The listing builds one solid part. Answer for the finished solid, in the listing's coordinates (mm). A direction names the side the tool comes from. Coordinates: 2 decimals unless noted, no trailing zeros. Order: outer loops, then holes, each group sorted by start corner. A loop starts at its lowest first (then second) coordinate and runs counter-clockwise, first axis right, second up. Notation, with made-up numbers: (68.5, -1) -> (119.5, -1) arc R5 cw to (119.5, 4) -> close; hole circle Ø8 at (70.5, 42.25). An arc over 180 degrees is marked (long way). Answer in a Markdown table with one row per item.
```python
from build123d import *

# Parameters (mm, degrees)
BOSS_EXTRUDE1_DEPTH = 11
CHAMFER1_SIZE       = 0.325


with BuildPart() as part:
    # Sketch1 → Boss-Extrude1 (new body)
    with BuildSketch(Plane(origin=(0, 0, 0), x_dir=(0, -1, 0), z_dir=(-1, 0, 0))):
        Polygon((2.886751346, 0), (1.443375673, 2.5), (-1.443375673, 2.5), (-2.886751346, 0), (-1.443375673, -2.5), (1.443375673, -2.5), align=None)
    extrude(amount=-BOSS_EXTRUDE1_DEPTH)

    # Sketch2 → Cut-Revolve1 (revolve, cut)
    with BuildSketch(Plane.XY, mode=Mode.PRIVATE) as cut_revolve1_sk:
        Polygon((0, 1.229375), (0, 0), (9.999979987, 0), (9.2902, 1.229375), (8.270625, 1.229375), (8, 1.5), (8, 1.229375), align=None)
    revolve(cut_revolve1_sk.sketch.rotate(Axis((0, 0, 0), (1, 0, 0)), 270), axis=Axis((0, 0, 0), (1, 0, 0)), mode=Mode.SUBTRACT)

    # Sketch3 → Revolve1 (revolve)
    with BuildSketch(Plane(origin=(0, 0, 0), x_dir=(-1, 0, 0), z_dir=(0, 0, -1)), mode=Mode.PRIVATE) as revolve1_sk:
        Polygon((-17, 1.5), (-17, 0), (-11, 0), (-11, 1.175), (-12.2, 1.175), (-12.2, 1.5), align=None)
    revolve(revolve1_sk.sketch.rotate(Axis((17, 0, 0), (-1, 0, 0)), 270), axis=Axis((17, 0, 0), (-1, 0, 0)))

    # Chamfer1
    chamfer1_edges = [part.edges().sort_by_distance(p)[0] for p in [
        (0, 0, 1.229375),
        (17, 0, -1.5),
    ]]
    chamfer(chamfer1_edges, length=CHAMFER1_SIZE)


solid = part.part
```
(1) Which of the six approach directions +Z, -Z, +X, -X, +Y, -Y give full straight-line access (tool end or side, diameter ignored) to faces 1 (the cylindrical face through (4.11, 1.22, 0.16)), 2 (the flat face through (11, -1, 1)), 3 (the flat face through (17, 0, 0)), 4 (the cylindrical face through (14.47, 0.45, 1.43))?
Check values:
| item | result |
|---|---|
| face 1 | -X |
| face 2 | none |
| face 3 | +Z, -Z, +X, +Y, -Y |
| face 4 | +X |
(2) A cutting plane is placed at A-A, the plane x = 3.5. Determine the outline of the cut face in (y, z), then the cut area to 3 significant figures.
Check values:
| item | result |
|---|---|
| outline | (-2.89, 0) -> (-1.44, -2.5) -> (1.44, -2.5) -> (2.89, 0) -> (1.44, 2.5) -> (-1.44, 2.5) -> close; hole circle Ø2.46 at (0, 0) |
| area | 16.9 mm² |
(3) A cutting plane is placed at B-B, the plane x = 10.25. Determine the outline of the cut face in (y, z), then the cut area to 3 significant figures.
Check values:
| item | result |
|---|---|
| outline | (-2.89, 0) -> (-1.44, -2.5) -> (1.44, -2.5) -> (2.89, 0) -> (1.44, 2.5) -> (-1.44, 2.5) -> close |
| area | 21.7 mm² |
(4) Find the intervals of material crossed by line 1 along X through (y, z) = (-1.6, 0.5); line 2 along Z through (x, y) = (8.5, -2.6); line 3 along Z through (x, y) = (13.25, -1.2), in increasing order. Write a range as from..to.
Check values:
| item | result |
|---|---|
| line 1 | 0..11 |
| line 2 | -0.5..0.5 |
| line 3 | -0.9..0.9 |
(5) A cutting plane is placed at C-C, the plane z = 2.25. Determine the outline of the cut face in (x, y), then the cut area to 3 significant figures.
Check values:
| item | result |
|---|---|
| outline | (0, -1.59) -> (11, -1.59) -> (11, 1.59) -> (0, 1.59) -> close |
| area | 34.9 mm² |
(6) Flat-ended cylindrical pins translate along their axes: pin 1 (2 mm diameter, centred on x = 9, y = -2.5, fed in from +Z); pin 2 (2 mm diameter, centred on x = 11.5, z = -2, fed in from +Y); pin 3 (1.5 mm diameter, centred on x = 15, y = 1, fed in from -Z). Find the tip coordinate at first contact, or state that the pin passes through.
Check values:
| item | result |
|---|---|
| pin 1 | z = 2.4 |
| pin 2 | y = 2.23 |
| pin 3 | z = -1.48 |
(7) For a pull along X with two mould halves and no side action, classify faces 5 (the cylindrical face through (11.61, 0.35, 1.12)), 6 (the conical face through (10, 0, 0)), 7 (the flat face through (5.423, -2.155, -1.267)) as released by +X, released by -X, zero draft, split by the parting line, or undercut.
Check values:
| item | result |
|---|---|
| face 5 | undercut |
| face 6 | released by -X |
| face 7 | zero draft |
(8) A cutting plane is placed at D-D, the plane y = -1.75. Determine the outline of the cut face in (x, z), then the cut area to 3 significant figures.
Check values:
| item | result |
|---|---|
| outline | (0, -1.97) -> (11, -1.97) -> (11, 1.97) -> (0, 1.97) -> close |
| area | 43.3 mm² |
